from build123d import *

# Parameters (mm, degrees)
SKETCH1_W           = 10
SKETCH1_H           = 2
SKETCH1_W_2         = 2
SKETCH1_H_2         = 5
SKETCH1_W_3         = 8.5
SKETCH1_H_3         = 13.5
BOSS_EXTRUDE1_DEPTH = 2


with BuildPart() as part:
    # Sketch1 → Boss-Extrude1 (new body)
    with BuildSketch(Plane.XY):
        Polygon((0, 0), (3, 0), (3, -2), (48, -2), (48, 0), (51, 0), (51, 12.5), (53, 12.5), (53, 17.5), (51, 17.5), (51, 49), (53, 49), (53, 54), (51, 54), (51, 87), (53, 87), (53, 92), (51, 92), (51, 106), (0, 106), (0, 92), (-2, 92), (-2, 87), (0, 87), (0, 54), (-2, 54), (-2, 49), (0, 49), (0, 17.5), (-2, 17.5), (-2, 12.5), (0, 12.5), align=None)
        with Locations((25.5, 31)):
            Rectangle(SKETCH1_W, SKETCH1_H, mode=Mode.SUBTRACT)
        with Locations((25.5, 74)):
            Rectangle(SKETCH1_W, SKETCH1_H, mode=Mode.SUBTRACT)
        with Locations((19, 52.5)):
            Rectangle(SKETCH1_W_2, SKETCH1_H_2, mode=Mode.SUBTRACT)
        with Locations((14.25, 13.25)):
            Rectangle(SKETCH1_W_3, SKETCH1_H_3, mode=Mode.SUBTRACT)
    extrude(amount=BOSS_EXTRUDE1_DEPTH)


solid = part.part
Geometry check sheet. Reference: the model listing, model coordinates, mm. A direction names the side the tool comes from. Give positions to 0.01 mm unless a question says otherwise; leave off trailing zeros. Write each loop counter-clockwise with the first axis right and the second up, starting at its lowest first coordinate (ties: lowest second). Pieces come first, ordered by that corner, then holes. Notation, with made-up numbers: (3, -29) - (62, -29) arc R21 cw to (62, 2) - close; hole circle Ø10 at (25.5, 27.25). An arc over 180 degrees is marked (long way). Put each result on its own line as item: value.
1. Sectioned sample at A-A, the plane z = 0.6. Give the number of separate pieces and of enclosed holes in the cut face, plus the area to 3 significant figures.
Ans:
separate pieces: 1
enclosed holes: 4
area: 5,390 mm²
2. Go/stop test with flat-tipped pins: pin 1 (0.6 mm diameter, centred on x = -1, z = 1, fed in from +Y); pin 2 (0.6 mm diameter, centred on x = 2, z = 1.5, fed in from -Y); pin 3 (1 mm diameter, centred on x = 52, z = 1, fed in from -Y). Record where each tip stops, or that it passes through.
Ans:
pin 1: stops at y = 92
pin 2: stops at y = 0
pin 3: stops at y = 12.5
3. Set-up check for faces 1 (the flat face through (52, 92, 1)), 2 (the flat face through (20, 52, 1)), 3 (the flat face through (-1, 54, 1)), 4 (the flat face through (51, 70, 1)): record each of +Z, -Z, +X, -X, +Y, -Y from which the full face is reachable in a straight line by a thin tool's end or side.
Ans:
face 1: +Z, -Z, +X, +Y
face 2: +Z, -Z
face 3: +Z, -Z, -X
face 4: +Z, -Z, +X
4. Sectioned sample at B-B, the plane y = 64.5. Enter the section's corners in (x, z), plus the area to 3 significant figures.
Ans:
outline: (0, 0) - (51, 0) - (51, 2) - (0, 2) - close
area: 102 mm²
5. Thickness scan on line 1 (Y direction, x = 15, z = 0.45); line 2 (Y direction, x = 21, z = 1.7); line 3 (X direction, y = 19, z = 0.5). Record the ranges inside material, lowest first.
Ans:
line 1: y = -2 to 6.5, 20 to 106
line 2: y = -2 to 30, 32 to 73, 75 to 106
line 3: x = 0 to 10, 18.5 to 51
6. Draft check along X on faces 5 (the flat face through (53, 89, 1)), 6 (the flat face through (18.5, 13, 1)), 7 (the flat face through (25, 53, 2)), 8 (the flat face through (3, -1, 1)). Enter one of: +X half, -X half, draft (parallel to the pull), parting line (faces both ways), or undercut.
Ans:
face 5: +X half
face 6: undercut
face 7: draft
face 8: -X half
